Geometry check sheet. Reference: the model listing, model coordinates, mm. A direction names the side the tool comes from. Give positions to 0.01 mm unless a question says otherwise; leave off trailing zeros. Write each loop counter-clockwise with the first axis right and the second up, starting at its lowest first coordinate (ties: lowest second). Pieces come first, ordered by that corner, then holes. Notation, with made-up numbers: M 35,-13 L 41,-13 A15 ccw 41,6 Z; hole C -26,74.5 d11. An arc over 180 degrees is marked long. One line per item, written item: value. Start each with the question number.
1. Cross-section at B-B on y = 2.75. Record the cut outline in (x, z).
2. Cross-section at C-C on z = -13.5. Record the cut outline in (x, y), then the cut area to 3 significant figures.
3. Cross-section at A-A on x = 0. Record the cut outline in (y, z).
4. Tool access check on faces 1 (the face through (-9, 1, 10.067)), 2 (the face through (-9, 1, 0)), 3 (the face through (0, -2.5, 0)). Record the directions out of +Z, -Z, +X, -X, +Y, -Y that give a thin tool (end or side, any length) a straight path to the whole face; none if there is none.
5. Cross-section at D-D on y = -0.75. Record the cut outline in (x, z), then the cut area to 3 significant figures.
6. Scan lines: line 1 (Z direction, x = 0, y = -7.25); line 2 (Y direction, x = -5, z = -12.5); line 3 (Z direction, x = 8, y = -7.5). Record each from-to range of solid material in increasing order.
7. Gauge pin test, flat ends, axial feed: pin 1 (4 mm diameter, centred on x = 0.5, z = -6.5, fed in from +Y); pin 2 (4.5 mm diameter, centred on x = -10, y = 2.5, fed in from -Z); pin 3 (4 mm diameter, centred on x = 11, y = 0.5, fed in from +Z). Record the tip position at first contact, or that the pin passes through.
8. Release check for a two-part mould opening along X. For faces 4 (the face through (-11, 5, 5)), 5 (the face through (-4.918, -6.198, -22.146)), 6 (the face through (-9.18, 1.92, 5.1)), 7 (the face through (-13.157, 2, 5)) record: pulls with the +X half, pulls with the -X half, needs draft (parallel to the pull), parting line crosses it, or undercut.
from build123d import *

# Parameters (mm, degrees)
F0_R     = 25.1852873168
F1_DEPTH = 10
F2_T     = -2.5
F3_W     = 5.0779422745
F3_H     = 10.067243129
F4_DEPTH = 5
F5_R     = 1
F7_D     = 3


with BuildPart() as f1:
    # F0 (on Front) → F1 (new body)
    with BuildSketch(Plane.XZ):
        Circle(F0_R)
    extrude(amount=F1_DEPTH)

    # F2
    f2_openings = [f1.faces().sort_by_distance(p)[0] for p in [
        (0, -10, 0),
    ]]
    offset(amount=F2_T, openings=f2_openings)

    # F3 (on face) → F4 (join)
    with BuildSketch(Plane(origin=(0, 0, 0), x_dir=(-1, 0, 0), z_dir=(0, 1, 0))):
        with Locations((10.6177399866, 5.0336215645)):
            Rectangle(F3_W, F3_H)
    extrude(amount=F4_DEPTH)

    # F5
    f5_edges = [f1.edges().sort_by_distance(p)[0] for p in [
        (-8.078769, 5, 5.033622),
        (-10.61774, 5, 0),
        (-13.156711, 5, 5.033622),
        (-10.61774, 5, 10.067243),
    ]]
    fillet(f5_edges, radius=F5_R)

    # F7 (through all)
    with Locations(Plane(origin=(0, 0, 0), x_dir=(1, 0, 0), z_dir=(0, 0, -1))):
        with Locations((-10.6769287959, -1.9884661306)):
            Hole(F7_D / 2)


solid = f1.part
Report:
1. outline: M -13.16,0 L -11.97,0 L -11.97,10.07 L -13.16,10.07 Z; M -9.38,0 L -8.08,0 L -8.08,10.07 L -9.38,10.07 Z
2. outline: M -21.26,-10 L -18.23,-10 L -18.23,-2.5 L 18.23,-2.5 L 18.23,-10 L 21.26,-10 L 21.26,0 L -21.26,0 Z
2. area: 152 mm^2
3. outline: M -10,-25.19 L 0,-25.19 L 0,25.19 L -10,25.19 L -10,22.69 L -2.5,22.69 L -2.5,-22.69 L -10,-22.69 Z
4. face 1: +Z, +X, -X, +Y
4. face 2: -Z, +X, -X, +Y
4. face 3: -Y
5. outline: C 0,0 d50.37
5. area: 1,990 mm^2
6. line 1: z = -25.19 to -22.69, 22.69 to 25.19
6. line 2: y = -2.5 to 0
6. line 3: z = -23.88 to -21.23, 21.23 to 23.88
7. pin 1: stops at y = 0
7. pin 2: stops at z = 0
7. pin 3: stops at z = 23.5
8. face 4: needs draft
8. face 5: undercut
8. face 6: undercut
8. face 7: pulls with the -X half
